CAD build for the part. Positions are in the model's coordinates, mm. A direction names the side the tool comes from. Round coordinates to 2 decimals unless told otherwise and drop trailing zeros. Write each loop counter-clockwise with the first axis right and the second up, starting at its lowest first coordinate (ties: lowest second). Pieces come first, ordered by that corner, then holes. Notation, with made-up numbers: (-38, 30.5) - (-29, 30.5) arc R21 ccw to (-29, 66.5) - close; hole circle Ø11 at (68.5, -13). An arc over 180 degrees is marked (long way). Answer in a Markdown table with one row per item.
```python
from build123d import *

# Parameters (mm, degrees)
EXTRUDE_1_DEPTH = 2
SKETCH_2_R      = 3
EXTRUDE_2_DEPTH = 6
SKETCH_3_R      = 4
SKETCH_3_R_2    = 2.5
EXTRUDE_3_DEPTH = 2


with BuildPart() as part:
    # ｽｹｯﾁ1 → 押し出し1 (new body)
    with BuildSketch(Plane(origin=(0, 0, 0), x_dir=(0, 0, -1), z_dir=(1, 0, 0))):
        with BuildLine():
            ThreePointArc((55, 16.483534558), (26.291521673, 12.27405221), (0, 0))
            Line((0, 0), (55, 0))
            Line((55, 0), (55, 16.483534558))
        make_face()
        with BuildLine():
            Line((55, 16.483534558), (55, 0))
            Line((55, 0), (110, 0))
            ThreePointArc((110, 0), (83.708478327, 12.27405221), (55, 16.483534558))
        make_face()
    extrude(amount=EXTRUDE_1_DEPTH)

    # ｽｹｯﾁ2 → 押し出し2 (add)
    with BuildSketch(Plane(origin=(2, 0, 0), x_dir=(0, 0, -1), z_dir=(1, 0, 0))):
        with Locations((23, 5)):
            Circle(SKETCH_2_R)
        with Locations((39, 10)):
            Circle(SKETCH_2_R)
        with Locations((55, 5)):
            Circle(SKETCH_2_R)
        with Locations((71, 10)):
            Circle(SKETCH_2_R)
        with Locations((87, 5)):
            Circle(SKETCH_2_R)
    extrude(amount=EXTRUDE_2_DEPTH)

    # ｽｹｯﾁ3 → 押し出し3 (add)
    # profile 1 of 5: a face of its own
    with BuildSketch(Plane(origin=(8, 0, 0), x_dir=(0, 0, -1), z_dir=(1, 0, 0))):
        with Locations((23, 5)):
            Circle(SKETCH_3_R)
        with Locations((23, 5)):
            Circle(SKETCH_3_R_2, mode=Mode.SUBTRACT)
    # profile 2 of 5: a face of its own
    with BuildSketch(Plane(origin=(8, 0, 0), x_dir=(0, 0, -1), z_dir=(1, 0, 0))):
        with Locations((39, 10)):
            Circle(SKETCH_3_R)
        with Locations((39, 10)):
            Circle(SKETCH_3_R_2, mode=Mode.SUBTRACT)
    # profile 3 of 5: a face of its own
    with BuildSketch(Plane(origin=(8, 0, 0), x_dir=(0, 0, -1), z_dir=(1, 0, 0))):
        with Locations((55, 5)):
            Circle(SKETCH_3_R)
        with Locations((55, 5)):
            Circle(SKETCH_3_R_2, mode=Mode.SUBTRACT)
    # profile 4 of 5: a face of its own
    with BuildSketch(Plane(origin=(8, 0, 0), x_dir=(0, 0, -1), z_dir=(1, 0, 0))):
        with Locations((71, 10)):
            Circle(SKETCH_3_R)
        with Locations((71, 10)):
            Circle(SKETCH_3_R_2, mode=Mode.SUBTRACT)
    # profile 5 of 5: a face of its own
    with BuildSketch(Plane(origin=(8, 0, 0), x_dir=(0, 0, -1), z_dir=(1, 0, 0))):
        with Locations((87, 5)):
            Circle(SKETCH_3_R)
        with Locations((87, 5)):
            Circle(SKETCH_3_R_2, mode=Mode.SUBTRACT)
    extrude(amount=EXTRUDE_3_DEPTH)


solid = part.part
```
Q1. Drill centre lines: line 1 (X direction, y = 13.75, z = -38); line 2 (Y direction, x = 8.6, z = -87); line 3 (Y direction, x = 9.65, z = -39). Where is each one in solid material? Low to high.
Computed:
| item | result |
|---|---|
| line 1 | x = 0 to 2, 8 to 10 |
| line 2 | y = 1 to 2.5, 7.5 to 9 |
| line 3 | y = 6 to 7.5, 12.5 to 14 |
Q2. Saw through at B-B on z = -87. List the corners of the cut face in (x, y).
Computed:
| item | result |
|---|---|
| outline | (0, 0) - (2, 0) - (2, 2) - (8, 2) - (8, 1) - (10, 1) - (10, 2.5) - (8, 2.5) - (8, 7.5) - (10, 7.5) - (10, 9) - (8, 9) - (8, 8) - (2, 8) - (2, 11.23) - (0, 11.23) - close |
Q3. 3-axis set-ups, long thin cutter, end or side, ignore diameter. For faces 5 (the flat face through (10, 7, -57)), 6 (the cylindrical face through (5, 5, -84)), 7 (the cylindrical face through (8.99, 4.04, -57.31)): which of +Z, -Z, +X, -X, +Y, -Y reach the whole face in a straight line?
Computed:
| item | result |
|---|---|
| face 5 | +Z, -Z, +X, +Y, -Y |
| face 6 | none |
| face 7 | +X |
Q4. Pull direction X, two halves, no side cores. Call faces 1 (the cylindrical face through (8.986, 6.201, -58.815)), 2 (the flat face through (0, 7, -54)), 3 (the cylindrical face through (5, 3.2, -20.6)), 4 (the flat face through (10, 3, -21)): released by +X, released by -X, zero draft, split by the parting line, or undercut.
Computed:
| item | result |
|---|---|
| face 1 | zero draft |
| face 2 | released by -X |
| face 3 | undercut |
| face 4 | released by +X |
Q5. Flat gauge pins, fed straight in: pin 1 (1 mm diameter, centred on x = 5.5, y = 10, fed in from +Z); pin 2 (1.5 mm diameter, centred on x = 3, z = -50, fed in from +Y); pin 3 (1 mm diameter, centred on x = 6, z = -73.5, fed in from -Y); pin 4 (4 mm diameter, centred on x = 5.5, y = 8.5, fed in from -Z). Where does each tip first touch, or does it go through?
Computed:
| item | result |
|---|---|
| pin 1 | stops at z = -36 |
| pin 2 | passes through |
| pin 3 | stops at y = 7.76 |
| pin 4 | stops at z = -89.6 |
Q6. Saw through at A-A on x = 3.25. List the corners of the cut face in (y, z).
Computed:
| item | result |
|---|---|
| outline | circle Ø6 at (5, -87); circle Ø6 at (5, -55); circle Ø6 at (5, -23); circle Ø6 at (10, -71); circle Ø6 at (10, -39) |
Q7. Saw through at D-D on z = -28. List the corners of the cut face in (x, y).
Computed:
| item | result |
|---|---|
| outline | (0, 0) - (2, 0) - (2, 12.77) - (0, 12.77) - close |
Q8. Saw through at C-C on z = -71. List the corners of the cut face in (x, y), then the cut area to 3 significant figures.
Computed:
| item | result |
|---|---|
| outline | (0, 0) - (2, 0) - (2, 7) - (8, 7) - (8, 6) - (10, 6) - (10, 7.5) - (8, 7.5) - (8, 12.5) - (10, 12.5) - (10, 14) - (8, 14) - (8, 13) - (2, 13) - (2, 15.2) - (0, 15.2) - close |
| area | 72.4 mm2 |
